Autodesk Inventor part; units mm, degrees
ref_plane "YZ Plane" through (0, 0, 0) normal (1, 0, 0) x (0, 1, 0)
ref_plane "XZ Plane" through (0, 0, 0) normal (0, 1, 0) x (-1, 0, 0)
ref_plane "XY Plane" through (0, 0, 0) normal (0, 0, 1) x (1, 0, 0)
sketch "Sketch1" plane through (0, 0, 0) normal (0, 1, 0) x (-1, 0, 0)
  line L0 (0, 0) -> (44.45, 0)
  line L1 (44.45, 0) -> (44.45, -25.4)
  line L2 (44.45, -25.4) -> (0, -25.4)
  line L3 (0, -25.4) -> (0, 0)
  circle A0 centre (12.7, -12.7) radius 3.2639
  circle A1 centre (31.75, -12.7) radius 3.2639
  point P0 (0, -12.7)
  dimension "d0" = 44.45
  dimension "d1" = 25.4
  dimension "d2" = 6.5278
  dimension "d3" = 19.05
  dimension "d4" = 12.7
  dimension "d5" = 12.7
extrude "Extrusion1" add sketch "Sketch1" along normal blind 6.35
sketch "Sketch2" plane through (0, 6.35, 0) normal (0, 1, 0) x (1, 0, 0)
  line L0 (0, 25.4) -> (-44.45, 25.4)
  line L1 (0, 0) -> (-6.35, 0)
  line L2 (-6.35, 0) -> (-6.35, 25.4)
  line L3 (-6.35, 25.4) -> (0, 25.4)
  line L4 (0, 25.4) -> (0, 0)
  dimension "d8" = 6.35
extrude "Extrusion2" add sketch "Sketch2" along normal blind 57.15
sketch "Sketch3" plane through (-6.35, 6.35, -25.4) normal (-1, 0, 0) x (0, 0, 1)
  circle A0 centre (12.7, 19.05) radius 2.4892
  circle A1 centre (12.7, 44.45) radius 2.4892
  line L0 (0, 0) -> (25.4, 0)
  line L1 (25.4, 0) -> (25.4, 57.15)
  circle A2 centre (12.7, 31.75) radius 2.4892
  point P0 (25.4, -6.35)
  dimension "d11" = 4.9784
  dimension "d12" = 4.9784
  dimension "d13" = 25.4
  dimension "d14" = 19.05
  dimension "d15" = 12.7
  dimension "d23" = 12.7
extrude "Extrusion3" cut sketch "Sketch3" against normal through all
sketch "Sketch4" plane through (-44.45, 0, 0) normal (0, 0, 1) x (1, 0, 0)
  line L0 (0, 6.35) -> (38.1, 6.35)
  line L1 (0, 0) -> (44.45, 0)
  line L2 (44.45, 0) -> (44.45, 63.5)
  line L3 (38.1, 63.5) -> (44.45, 63.5)
  line L4 (38.1, 6.35) -> (38.1, 63.5)
  line L5 (0, 6.35) -> (38.1, 6.35)
  line L6 (0, 0) -> (0, 6.35)
  line L7 (0, 6.35) -> (38.1, 63.5)
  line L8 (44.45, 63.5) -> (44.45, 0)
  line L9 (0, 0) -> (0, 6.35)
  line L10 (44.45, 0) -> (0, 0)
  line L11 (38.1, 63.5) -> (44.45, 63.5)
extrude "Extrusion4" add sketch "Sketch4" against normal blind 3.175 contours L7 L4 L0
sketch "Sketch5" plane through (0, 0, -25.4) normal (0, 0, -1) x (-1, 0, 0)
  line L0 (0, 0) -> (44.45, 0)
  line L1 (44.45, 0) -> (44.45, 6.35)
  line L2 (6.35, 6.35) -> (44.45, 6.35)
  line L3 (6.35, 6.35) -> (6.35, 63.5)
  line L4 (0, 63.5) -> (6.35, 63.5)
  line L5 (0, 0) -> (0, 63.5)
  line L6 (44.45, 6.35) -> (44.45, 0)
  line L7 (0, 0) -> (44.45, 0)
  line L8 (44.45, 6.35) -> (6.35, 63.5)
  line L9 (0, 0) -> (0, 63.5)
  line L10 (6.35, 63.5) -> (0, 63.5)
  line L11 (0, 63.5) -> (0, 0)
extrude "Extrusion5" add sketch "Sketch5" against normal blind 3.175
fillet "Fillet1" radius 6.35 2 edges at (-44.45, 3.175, -25.4) (-44.45, 3.175, 0)
properties part number "INDX_025_backshuffleBracket" material "ABS Plastic"
The listing builds one solid part. Answer for the finished solid, in the listing's coordinates (mm). A direction names the side the tool comes from. Round coordinates to 2 decimals unless told otherwise and drop trailing zeros. Loops run counter-clockwise (first coordinate to the right, second up) from the corner with the lowest first, then second, coordinate; pieces in that order, holes last. Notation, with made-up numbers: (-39.75, 33.25) - (13.25, 33.25) arc R28 ccw to (13.25, 69.25) - close; hole circle Ø11 at (68.25, -32). An arc over 180 degrees is marked (long way). Return JSON: item names as keys, results as strings. Group by question number.
1. Consider probe 1 along Y at (x, z) = (-4.25, -12.7); probe 2 along Z at (x, y) = (-31, 24) (3 decimals); probe 3 along X at (y, z) = (15.5, -5.75). Determine where each line is inside the solid, lowest interval first.
2. The part is cut by section C-C on x = -3. Determine the outline of the cut face in (y, z).
3. Which of the six approach directions +Z, -Z, +X, -X, +Y, -Y give full straight-line access (tool end or side, diameter ignored) to faces 1 (the cylindrical face through (-3.219, 35.892, -11.551)), 2 (the flat face through (-6.35, 35, -13))?
4. The part is cut by section A-A on x = -31.75. Determine the outline of the cut face in (y, z) (3 decimals).
5. Each of these flat-tipped pins is pushed along its axis until it touches: P1, Ø12, axis at y = 21, z = -13, coming from the -X side; P2, Ø8.5, axis at x = -31.75, z = -12.7, coming from the +Y side. Where does it stop, or does it pass through?
6. The part is cut by section D-D on y = 38.1. Determine the outline of the cut face in (x, z) (3 decimals).
7. The mould has two halves that part along Z. Classify faces 3 (the flat face through (-21, 23, -3.175)), 4 (the flat face through (0, 31, -13)), 5 (the flat face through (-15, 25, 0)): pulls with the +Z half, pulls with the -Z half, needs draft (parallel to the pull), parting line crosses it, or undercut.
8. The part is cut by section B-B on z = -12.7. Determine the outline of the cut face in (x, y).
Resolved:
{
 "1": {"probe 1": "y = 0 to 22.91, 27.89 to 35.61, 40.59 to 48.31, 53.29 to 63.5", "probe 2": "z = -25.4 to -22.225, -3.175 to 0", "probe 3": "x = -6.35 to 0"},
 "2": {"outline": "(0, -25.4) - (63.5, -25.4) - (63.5, 0) - (0, 0) - close; hole circle Ø4.98 at (25.4, -12.7); hole circle Ø4.98 at (38.1, -12.7); hole circle Ø4.98 at (50.8, -12.7)"},
 "3": {"face 1": "+X, -X", "face 2": "-X, +Y"},
 "4": {"outline": "(0, -25.4) - (25.4, -25.4) - (25.4, -22.225) - (6.35, -22.225) - (6.35, -15.964) - (0, -15.964) - close; (0, -9.436) - (6.35, -9.436) - (6.35, -3.175) - (25.4, -3.175) - (25.4, 0) - (0, 0) - close"},
 "5": {"P1": "stops at x = -6.35", "P2": "stops at y = 6.35"},
 "6": {"outline": "(-23.283, -25.4) - (0, -25.4) - (0, -15.189) - (-6.35, -15.189) - (-6.35, -22.225) - (-23.283, -22.225) - close; (-23.283, -3.175) - (-6.35, -3.175) - (-6.35, -10.211) - (0, -10.211) - (0, 0) - (-23.283, 0) - close"},
 "7": {"face 3": "undercut", "face 4": "needs draft", "face 5": "pulls with the +Z half"},
 "8": {"outline": "(-44.45, 0) - (-35.01, 0) - (-35.01, 6.35) - (-44.45, 6.35) - close; (-28.49, 0) - (-15.96, 0) - (-15.96, 6.35) - (-28.49, 6.35) - close; (-9.44, 0) - (0, 0) - (0, 22.91) - (-6.35, 22.91) - (-6.35, 6.35) - (-9.44, 6.35) - close; (-6.35, 27.89) - (0, 27.89) - (0, 35.61) - (-6.35, 35.61) - close; (-6.35, 40.59) - (0, 40.59) - (0, 48.31) - (-6.35, 48.31) - close; (-6.35, 53.29) - (0, 53.29) - (0, 63.5) - (-6.35, 63.5) - close"}
}
